Build history of the part. All positions in model axes, mm. A direction names the side the tool comes from. Give positions to 0.01 mm unless a question says otherwise; leave off trailing zeros. Write each loop counter-clockwise with the first axis right and the second up, starting at its lowest first coordinate (ties: lowest second). Pieces come first, ordered by that corner, then holes. Notation, with made-up numbers: M 19,6 L 31,6 A9 ccw 31,10 Z; hole C 26,24 d9. An arc over 180 degrees is marked long. Return JSON: item names as keys, results as strings. Group by question number.
Q1. Band-saw the part on A-A, the plane x = 0. Give the cut face in (y, z), then the cut area to 4 significant figures.
Q2. Band-saw the part on D-D, the plane z = 44. Give the cut face in (x, y).
Q3. Band-saw the part on C-C, the plane x = 63. Give the cut face in (y, z).
Q4. Band-saw the part on B-B, the plane y = -12.5. Give the cut face in (x, z).
Q5. Wall check: probe 1 along Y at (x, z) = (0, 3.5); probe 2 along Z at (x, y) = (-57, -113.5); probe 3 along Y at (x, z) = (-69.5, 11.5). Give the ranges that are in metal, low to high.
Q6. Flat gauge pins, fed straight in: pin 1 Ø1 at (x, z) = (70.5, 58) entering from -Y; pin 2 Ø1.5 at (y, z) = (-9.5, 47.5) entering from +X; pin 3 Ø8 at (x, y) = (28.5, -29) entering from +Z. Where does each tip first touch, or does it go through?
Q7. Tool access for faces 4 (the cylindrical face through (-1.856, -130.646, 53.225)), 5 (the flat face through (-20, -45, -8.78)): list every direction of +Z, -Z, +X, -X, +Y, -Y with a clear straight run to the whole face (end or side of a thin tool).
Q8. Pull direction Y, two halves, no side cores. Call faces 1 (the cylindrical face through (-1.11, 37.21, 53.22)), 2 (the flat face through (-65, -9, 65.747)), 3 (the cylindrical face through (28.957, 45.166, 15.44)): +Y half, -Y half, draft (parallel to the pull), parting line (faces both ways), or undercut.
from build123d import *

# Parameters (mm, degrees)
F0_W           = 96.4018628001
F0_H           = 49.1270134225
F2_DEPTH       = 25.4
F3_R           = 96.4018628001
F3_R_2         = 8.561445451
F4_DEPTH       = 25.4
F6_D           = 6.7564
F6_CSINK_D     = 13.4874
F6_CSINK_ANGLE = 82


with BuildPart() as f1:
    # F0 (on Right) → F1 (revolve)
    with BuildSketch(Plane.YZ):
        with Locations((1.4167837799, 15.7836410217)):
            Rectangle(F0_W, F0_H)
    revolve(axis=Axis((0, -46.7841476202, 15.7836410217), (0, 0, -1)))

    # F2 (add): a face of the model
    f2_faces = [f1.faces().sort_by_distance(p)[0] for p in [
        (0, -46.7841476202, 40.347147733),
    ]]
    extrude(f2_faces, amount=F2_DEPTH)

    # F3 (on face) → F4 (cut)
    with BuildSketch(Plane.XY.offset(65.747147733)):
        with Locations((0, -46.7841476202)):
            Circle(F3_R)
        with Locations((-65.3880895687, -84.5359787345)):
            Circle(F3_R_2, mode=Mode.SUBTRACT)
        with Locations((0, -122.2878098488)):
            Circle(F3_R_2, mode=Mode.SUBTRACT)
        with Locations((65.3880895687, -84.5359787345)):
            Circle(F3_R_2, mode=Mode.SUBTRACT)
        with Locations((-65.3880895687, -9.0323165059)):
            Circle(F3_R_2, mode=Mode.SUBTRACT)
        with Locations((65.3880895687, -9.0323165059)):
            Circle(F3_R_2, mode=Mode.SUBTRACT)
        with Locations((0, 28.7195146084)):
            Circle(F3_R_2, mode=Mode.SUBTRACT)
    extrude(amount=-F4_DEPTH, mode=Mode.SUBTRACT)

    # F6 (through all)
    with Locations(Plane.XY.offset(40.347147733)):
        with Locations((0, -46.7841476202)):
            CounterSinkHole(F6_D / 2, F6_CSINK_D / 2, counter_sink_angle=F6_CSINK_ANGLE)


solid = f1.part
From the geometry:
{
 "1": {"outline": "M -143.19,-8.78 L -50.16,-8.78 L -50.16,36.48 L -53.53,40.35 L -113.73,40.35 L -113.73,65.75 L -130.85,65.75 L -130.85,40.35 L -143.19,40.35 Z; M -43.41,-8.78 L 49.62,-8.78 L 49.62,40.35 L 37.28,40.35 L 37.28,65.75 L 20.16,65.75 L 20.16,40.35 L -40.04,40.35 L -43.41,36.48 Z", "area": "10,000 mm^2"},
 "2": {"outline": "C -65.39,-84.54 d17.12; C -65.39,-9.03 d17.12; C 0,-122.29 d17.12; C 0,28.72 d17.12; C 65.39,-84.54 d17.12; C 65.39,-9.03 d17.12"},
 "3": {"outline": "M -119.75,-8.78 L 26.18,-8.78 L 26.18,40.35 L -0.81,40.35 L -0.81,65.75 L -17.25,65.75 L -17.25,40.35 L -76.31,40.35 L -76.31,65.75 L -92.76,65.75 L -92.76,40.35 L -119.75,40.35 Z"},
 "4": {"outline": "M -90.1,-8.78 L 90.1,-8.78 L 90.1,40.35 L 73.22,40.35 L 73.22,65.75 L 57.56,65.75 L 57.56,40.35 L -57.56,40.35 L -57.56,65.75 L -73.22,65.75 L -73.22,40.35 L -90.1,40.35 Z"},
 "5": {"probe 1": "y = -143.19 to -50.16, -43.41 to 49.62", "probe 2": "z = -8.78 to 40.35", "probe 3": "y = -113.59 to 20.02"},
 "6": {"pin 1": "stops at y = -91.75", "pin 2": "stops at x = 73.95", "pin 3": "stops at z = 40.35"},
 "7": {"face 4": "+Z", "face 5": "-Z, +X, -X, +Y, -Y"},
 "8": {"face 1": "undercut", "face 2": "draft", "face 3": "parting line"}
}
